Print and shaded views of the part. All mm, measured from the part's lowest x, y and z. A direction names the side the tool comes from. Give positions to 0.01 mm unless a question says otherwise; leave off trailing zeros. Loops run counter-clockwise (first coordinate to the right, second up) from the corner with the lowest first, then second, coordinate; pieces in that order, holes last.
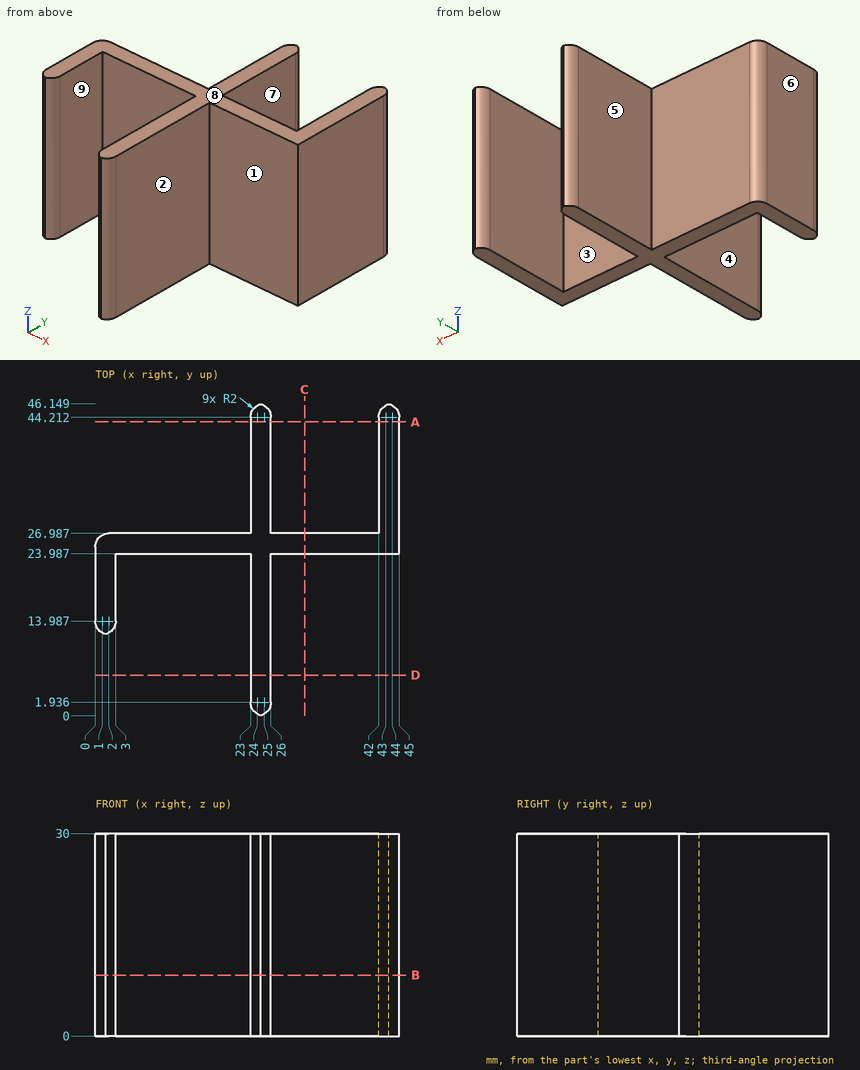
1. Saw through at D-D, the plane y = 6. List the corners of the cut face in (x, z).
Responses:
outline: (23, 0) - (26, 0) - (26, 30) - (23, 30) - close
2. Pull direction X, two halves, no side cores. Call the marked faces 1, 2, 3 and 4: released by +X, released by -X, zero draft, split by the parting line, or undercut.
Responses:
face 1: zero draft
face 2: released by +X
face 3: undercut
face 4: undercut
3. Tool access for the marked faces 5, 6, 7, 8 and 9: list every direction of +Z, -Z, +X, -X, +Y, -Y with a clear straight run to the whole face (end or side of a thin tool).
Responses:
face 5: +Z, -Z, -X, +Y
face 6: +Z, -Z, -X, +Y, -Y
face 7: +Z, -Z, +Y
face 8: +Z, +X, -X, +Y, -Y
face 9: +Z, -Z, -Y
4. Saw through at A-A, the plane y = 43.5. List the corners of the cut face in (x, z), and give its area (3 significant figures).
Responses:
outline: (23, 0) - (26, 0) - (26, 30) - (23, 30) - close; (42, 0) - (45, 0) - (45, 30) - (42, 30) - close
area: 180 mm2
5. Saw through at B-B, the plane z = 9. List the corners of the cut face in (x, y).
Responses:
outline: (0, 13.99) arc R2 ccw to (1.5, 12.05) arc R2 ccw to (3, 13.99) - (3, 23.99) - (23, 23.99) - (23, 1.94) arc R2 ccw to (24.5, 0) arc R2 ccw to (26, 1.94) - (26, 23.99) - (45, 23.99) - (45, 44.21) arc R2 ccw to (43.5, 46.15) arc R2 ccw to (42, 44.21) - (42, 26.99) - (26, 26.99) - (26, 44.21) arc R2 ccw to (24.5, 46.15) arc R2 ccw to (23, 44.21) - (23, 26.99) - (2, 26.99) arc R2 ccw to (0, 24.99) - close
6. Probe line 1 along X through (y, z) = (18.5, 4.25); line 2 along X through (y, z) = (33.5, 23.25); line 3 along Y through (x, z) = (8.5, 1). List the from-to ranges inside material, lowest first.
Responses:
line 1: x = 0 to 3, 23 to 26
line 2: x = 23 to 26, 42 to 45
line 3: y = 23.99 to 26.99
7. Saw through at C-C, the plane x = 31. List the corners of the cut face in (y, z).
Responses:
outline: (23.99, 0) - (26.99, 0) - (26.99, 30) - (23.99, 30) - close
8. Drop flat-ended pins along their axis: pin 1 (6.5 mm diameter, centred on x = 10, z = 15.5, fed in from +Y); pin 2 (8.5 mm diameter, centred on y = 34, z = 13.5, fed in from -X); pin 3 (2 mm diameter, centred on x = 37.5, z = 5, fed in from -Y); pin 4 (6 mm diameter, centred on x = 11.5, y = 19.5, fed in from +Z). Give the stop position or say it passes through.
Responses:
pin 1: stops at y = 26.99
pin 2: stops at x = 23
pin 3: stops at y = 23.99
pin 4: passes through
